Could you check a few things on this model? Use its own coordinates, in mm. Face numbers are marked on the shaded views. A direction names the side the tool comes from. Round coordinates to 2 decimals unless told otherwise and drop trailing zeros. Loops run counter-clockwise (first coordinate to the right, second up) from the corner with the lowest first, then second, coordinate; pieces in that order, holes last. Notation, with made-up numbers: (-19.75, -29) -> (7.25, -29) arc R20 ccw to (7.25, -10) -> close; hole circle Ø5 at (-26.5, 33.25). An arc over 180 degrees is marked (long way). One line per item, written item: value.
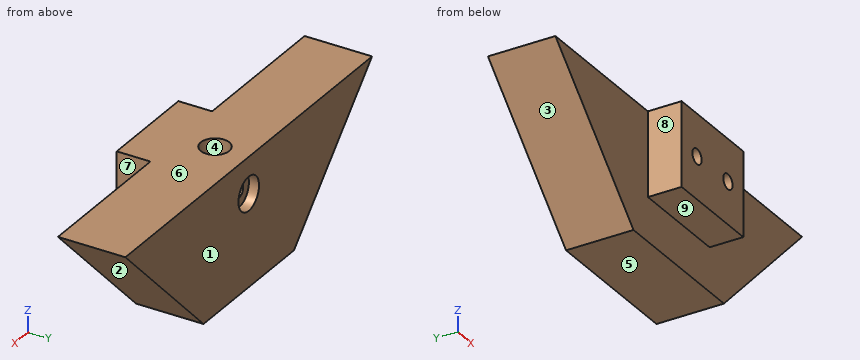
from build123d import *

# Parameters (mm, degrees)
BOSS_EXTRUDE1_DEPTH = 20
SKETCH2_R           = 5
CUT_EXTRUDE1_DEPTH  = 3
SKETCH3_R           = 2.25
CUT_EXTRUDE2_DEPTH  = 10
SKETCH4_R           = 4.25
CUT_EXTRUDE3_DEPTH  = 20
SKETCH5_W           = 30
SKETCH5_H           = 25
BOSS_EXTRUDE2_DEPTH = 10
SKETCH6_R           = 2.25
CUT_EXTRUDE7_DEPTH  = 10


with BuildPart() as part:
    # Sketch1 → Boss-Extrude1 (new body)
    with BuildSketch(Plane(origin=(0, 0, 0), x_dir=(1, 0, 0), z_dir=(0, 1, 0))):
        Polygon((0, 0), (60, 0), (22, 38), (0, 38), (-22, 38), (-60, 0), align=None)
    extrude(amount=BOSS_EXTRUDE1_DEPTH)

    # Sketch2 → Cut-Extrude1 (cut)
    with BuildSketch(Plane(origin=(0, 20, 0), x_dir=(1, 0, 0), z_dir=(0, 1, 0))):
        with Locations(Location((0, 10.75, 0), (0, 0, 270))):
            Circle(SKETCH2_R)
    extrude(amount=-CUT_EXTRUDE1_DEPTH, mode=Mode.SUBTRACT)

    # Sketch3 → Cut-Extrude2 (cut)
    with BuildSketch(Plane(origin=(0, 20, 0), x_dir=(1, 0, 0), z_dir=(0, 1, 0))):
        with Locations(Location((0, 10.75, 0), (0, 0, 270))):
            Circle(SKETCH3_R)
    extrude(amount=-CUT_EXTRUDE2_DEPTH, mode=Mode.SUBTRACT)

    # Sketch4 → Cut-Extrude3 (cut)
    with BuildSketch(Plane.XY):
        with Locations((0, 10)):
            Circle(SKETCH4_R)
    extrude(amount=-CUT_EXTRUDE3_DEPTH, mode=Mode.SUBTRACT)

    # Sketch5 → Boss-Extrude2 (add)
    with BuildSketch(Plane.XZ):
        with Locations((0, -12.5)):
            Rectangle(SKETCH5_W, SKETCH5_H)
    extrude(amount=BOSS_EXTRUDE2_DEPTH)

    # Sketch6 → Cut-Extrude7 (cut)
    with BuildSketch(Plane.XZ.offset(10)):
        with Locations(Location((-7.5, -12.5, 0), (0, 0, 270))):
            Circle(SKETCH6_R)
        with Locations(Location((7.5, -12.5, 0), (0, 0, 270))):
            Circle(SKETCH6_R)
    extrude(amount=-CUT_EXTRUDE7_DEPTH, mode=Mode.SUBTRACT)


solid = part.part
(1) For the marked faces 5, 6, 7, 8 and 9, which set-ups out of +Z, -Z, +X, -X, +Y, -Y let a thin tool reach every point of the face, with its end or its side?
Recorded:
face 5: -Z, +X, -X, +Y, -Y
face 6: +Z, +X, -X, +Y, -Y
face 7: +Z, -Z, +X, -Y
face 8: +Z, -Z, -X, -Y
face 9: -Z, +X, -X, -Y
(2) If we section it at A-A, the plane y = 18.25: Please give me the cut outline in (x, z).
Recorded:
outline: (-60, 0) -> (-22, -38) -> (22, -38) -> (60, 0) -> close; hole circle Ø10 at (0, -10.75)
(3) If we section it at C-C, the plane y = -2: Please give me the cut outline in (x, z).
Recorded:
outline: (-15, -25) -> (15, -25) -> (15, 0) -> (-15, 0) -> close; hole circle Ø4.5 at (-7.5, -12.5); hole circle Ø4.5 at (7.5, -12.5)
(4) Thinking about a two-plate mould opening in X: for the marked faces 1, 2, 3 and 4, which applies, released by +X, released by -X, zero draft, split by the parting line, or undercut?
Recorded:
face 1: zero draft
face 2: released by +X
face 3: released by -X
face 4: undercut
(5) If we section it at D-D, the plane y = 8: Please give me the cut outline in (x, z).
Recorded:
outline: (-60, 0) -> (-22, -38) -> (22, -38) -> (60, 0) -> (3.75, 0) -> (3.75, -20) -> (-3.75, -20) -> (-3.75, 0) -> close
(6) I'm going to push flat-ended pins straight in: pin 1 Ø4 at (x, z) = (-7.5, -12.5) entering from -Y; pin 2 Ø8 at (y, z) = (-6, -25) entering from -X; pin 3 Ø6 at (y, z) = (-0.5, -4) entering from -X. Where does each tip first touch, or does it pass through?
Recorded:
pin 1: y = 0
pin 2: x = -15
pin 3: x = -58.96
(7) If we section it at B-B, the plane x = -7.5: Please give me the cut outline in (y, z).
Recorded:
outline: (-10, -25) -> (0, -25) -> (0, -38) -> (20, -38) -> (20, 0) -> (-10, 0) -> (-10, -10.25) -> (0, -10.25) -> (0, -14.75) -> (-10, -14.75) -> close
(8) If I drill on L1, parallel to X at y = -6.75, z = -12.5; L2, parallel to Z at x = 0, y = 15; L3, parallel to Y at x = -19.5, z = -33, over which ranges is the centre line in solid material (lowest first)?
Recorded:
L1: -15 to -9.75, -5.25 to 5.25, 9.75 to 15
L2: -38 to -13, -8.5 to 0
L3: 0 to 20
